Here's how the part is built. I have some questions about the finished solid (model axes, mm). A direction names the side the tool comes from. Coordinates: 2 decimals unless noted, no trailing zeros. Loops run counter-clockwise (first coordinate to the right, second up) from the corner with the lowest first, then second, coordinate; pieces in that order, holes last. Notation, with made-up numbers: M 62.5,-37.75 L 121.5,-37.75 A9 cw 121.5,-21.75 Z; hole C 86.25,-4.5 d1. An arc over 180 degrees is marked long. Use one line per item in the form item = value. Start each with the question number.
(1) On a 3-axis mill with a long thin cutter (end or side, diameter ignored), from which of +Z, -Z, +X, -X, +Y, -Y can I reach the whole of each face in a straight line? I mean faces 1 (the flat face through (14, 0, -1.25)), 2 (the cylindrical face through (13.42, 1.02, 1.01)), 3 (the cylindrical face through (13.42, 1.01, -1.02)), 4 (the cylindrical face through (13.76, -1.01, 1.02)), 5 (the flat face through (14, 1.25, 0)). Say none if no direction works.
(2) Will these pins go through, and if not, where does the flat tip stop? P1, Ø1, axis at x = 18.5, z = 0, coming from the -Y side; P2, Ø1.5, axis at x = 8, y = -1, coming from the -Z side; P3, Ø0.7, axis at x = 12, z = 0, coming from the +Y side; P4, Ø1.5, axis at y = -0.5, z = -1.5, coming from the -X side.
(3) Imagine slicing it at C-C, the plane z = 0.1. Please give me the cut outline in (x, y), and give its area (3 significant figures).
(4) Thinking about a two-plate mould opening in X: for faces 6 (the cylindrical face through (13.76, -1.01, -1.02)), 7 (the flat face through (28, 0, -1.6)), which applies, +X half, -X half, draft (parallel to the pull), parting line (faces both ways), or undercut?
(5) Imagine slicing it at A-A, the plane y = 0. Please give me the cut outline in (x, z), and give its area (3 significant figures).
(6) Imagine slicing it at D-D, the plane x = 8.5. Please give me the cut outline in (y, z), and give its area (3 significant figures).
(7) Please list where these lines run through material, in increasing order: L1, parallel to Y at x = 0, z = -0.4; L2, parallel to X at y = 0.2, z = 0.3; L3, parallel to X at y = 0.1, z = -0.8.
(8) Imagine slicing it at B-B, the plane x = 0. Please give me the cut outline in (y, z).
```python
from build123d import *

# Parameters (mm, degrees)
SKETCH_1_R                       = 2
SKETCH_1_R_2                     = 0.36
EXTRUDE_1_DEPTH                  = 1.6
SKETCH_1_R_3                     = 0.42
EXTRUDE_1_2_DEPTH                = 1.6
EXTRUDE_2_REACH                  = 28.306
EXTRUDE_2_END_RADIUS             = 2
SKETCH_2_W                       = 2.5
SKETCH_2_H                       = 2.5
EXTRUDE_2_DIRECTION_2_REACH      = 28.306
EXTRUDE_2_DIRECTION_2_END_RADIUS = 2
CHAMFER_1_SIZE                   = 0.1
FILLET_1_R                       = 0.8


with BuildPart() as part:
    # Sketch 1 → Extrude 1 (new, symmetric)
    with BuildSketch(Plane.XY):
        Circle(SKETCH_1_R)
        Circle(SKETCH_1_R_2, mode=Mode.SUBTRACT)
    extrude(amount=EXTRUDE_1_DEPTH, both=True)



with BuildPart() as body_2:
    # Sketch 1 → Extrude 1 2 (new, symmetric)
    with BuildSketch(Plane.XY):
        with Locations((27.180718048, 0)):
            Circle(SKETCH_1_R)
        with Locations((27.180718048, 0)):
            Circle(SKETCH_1_R_3, mode=Mode.SUBTRACT)
    extrude(amount=EXTRUDE_1_2_DEPTH, both=True)


with BuildPart() as part_1:
    add(part.part)

    add(body_2.part)  # Extrude 2 merges body 2
    # Extrude 2: up to this cylinder (the profile starts outside it)
    extrude_2_end = Plane(origin=(27.180718048, 0, 0), z_dir=(0, 0, -1)) * Cylinder(EXTRUDE_2_END_RADIUS, 61.612, mode=Mode.PRIVATE)
    # Sketch 2 → Extrude 2 (add, up to the surface)
    with BuildSketch(Plane(origin=(3, 0, 0), x_dir=(0, 0, -1), z_dir=(1, 0, 0)), mode=Mode.PRIVATE) as extrude_2_sk1:
        Rectangle(SKETCH_2_W, SKETCH_2_H)
    extrude_2_tool1 = extrude(extrude_2_sk1.sketch, amount=EXTRUDE_2_REACH, mode=Mode.PRIVATE) - extrude_2_end
    add(extrude_2_tool1.solids().sort_by_distance((3, 0, 0))[0])

    # Extrude 2 direction 2: up to this cylinder (the profile starts outside it)
    extrude_2_direction_2_end = Plane(origin=(0, 0, 0), z_dir=(0, 0, -1)) * Cylinder(EXTRUDE_2_DIRECTION_2_END_RADIUS, 61.612, mode=Mode.PRIVATE)
    # Sketch 2 → Extrude 2 direction 2 (add, up to the surface)
    with BuildSketch(Plane(origin=(3, 0, 0), x_dir=(0, 0, -1), z_dir=(1, 0, 0)), mode=Mode.PRIVATE) as extrude_2_direction_2_sk1:
        Rectangle(SKETCH_2_W, SKETCH_2_H)
    extrude_2_direction_2_tool1 = extrude(extrude_2_direction_2_sk1.sketch, amount=-EXTRUDE_2_DIRECTION_2_REACH, mode=Mode.PRIVATE) - extrude_2_direction_2_end
    add(extrude_2_direction_2_tool1.solids().sort_by_distance((3, 0, 0))[0])

    # Chamfer 1
    chamfer_1_edges = [part_1.edges().sort_by_distance(p)[0] for p in [
        (26.760718048, 0, -1.6),
        (26.760718048, 0, 1.6),
        (-0.36, 0, -1.6),
        (-0.36, 0, 1.6),
    ]]
    chamfer(chamfer_1_edges, length=CHAMFER_1_SIZE)

    # Fillet 1
    fillet_1_edges = [part_1.edges().sort_by_distance(p)[0] for p in [
        (13.590359024, -1.25, 1.25),
        (13.590359024, -1.25, -1.25),
        (13.590359024, 1.25, -1.25),
        (13.590359024, 1.25, 1.25),
    ]]
    fillet(fillet_1_edges, radius=FILLET_1_R)


solid = part_1.part
```
Answer:
q1.face_1 = -Z, +Y, -Y
q1.face_2 = +Z, +Y
q1.face_3 = -Z, +Y
q1.face_4 = +Z, -Y
q1.face_5 = +Z, -Z, +Y
q2.P1 = -1.25
q2.P2 = -1.25
q2.P3 = 1.25
q2.P4 = -2
q3.outline = M 1.56,-1.25 L 25.62,-1.25 A2 ccw long 25.62,1.25 L 1.56,1.25 A2 ccw long Z; hole C 0,0 d0.72; hole C 27.18,0 d0.84
q3.area = 82.8 mm²
q4.face_6 = undercut
q4.face_7 = draft
q5.outline = M -2,-1.6 L -0.46,-1.6 L -0.36,-1.5 L -0.36,1.5 L -0.46,1.6 L -2,1.6 Z; M 0.36,-1.5 L 0.46,-1.6 L 2,-1.6 L 2,-1.25 L 25.18,-1.25 L 25.18,-1.6 L 26.66,-1.6 L 26.76,-1.5 L 26.76,1.5 L 26.66,1.6 L 25.18,1.6 L 25.18,1.25 L 2,1.25 L 2,1.6 L 0.46,1.6 L 0.36,1.5 Z; M 27.6,-1.5 L 27.7,-1.6 L 29.18,-1.6 L 29.18,1.6 L 27.7,1.6 L 27.6,1.5 Z
q5.area = 78.5 mm²
q6.outline = M -1.25,-0.45 A0.8 ccw -0.45,-1.25 L 0.45,-1.25 A0.8 ccw 1.25,-0.45 L 1.25,0.45 A0.8 ccw 0.45,1.25 L -0.45,1.25 A0.8 ccw -1.25,0.45 Z
q6.area = 5.70 mm²
q7.L1 = -2 to -0.36, 0.36 to 2
q7.L2 = -1.99 to -0.3, 0.3 to 26.81, 27.55 to 29.17
q7.L3 = -2 to -0.35, 0.35 to 26.77, 27.59 to 29.18
q8.outline = M -2,-1.6 L -0.46,-1.6 L -0.36,-1.5 L -0.36,1.5 L -0.46,1.6 L -2,1.6 Z; M 0.36,-1.5 L 0.46,-1.6 L 2,-1.6 L 2,1.6 L 0.46,1.6 L 0.36,1.5 Z
